For this review, take the finished solid that the model builds, in its own axes (mm). A direction names the side the tool comes from. Coordinates: 2 decimals unless noted, no trailing zeros. Order: outer loops, then holes, each group sorted by start corner. A loop starts at its lowest first (then second) coordinate and runs counter-clockwise, first axis right, second up. Notation, with made-up numbers: (51, 12.25) -> (84, 12.25) arc R33 cw to (84, 45.25) -> close; hole circle Ø1 at (-26.5, -34.5). An arc over 180 degrees is marked (long way). Return JSON: item names as keys, results as strings. Group by question number.
Item 1: Draft analysis for pull direction Z (two halves, no side actions). For faces 3 (the cylindrical face through (-276.009, 3.694, -370.875)), 4 (the flat face through (-111.6, 7.83, -280.08)), 5 (the flat face through (-258, 8, 0)), state which applies: +Z half, -Z half, draft (parallel to the pull), parting line (faces both ways), or undercut.
Item 2: For line 1 along Y through (x, z) = (-252, -378) (3 decimals); line 2 along Z through (x, y) = (-79, 7.75); line 3 along Z through (x, y) = (-194, 1.25), list the stretches that pass through material, from the lowest coordinate up.
Item 3: Take a section at D-D (x = -396.5). Write out the cut boundary in (y, z) (3 decimals).
Item 4: Take a section at B-B (x = -91.5). Write out the cut boundary in (y, z) (3 decimals).
Item 5: Take a section at C-C (z = -192). Write out the cut boundary in (x, y) (3 decimals).
Item 6: Machinability: for faces 1 (the cylindrical face through (-438.72, 3.69, -70.96)), 2 (the flat face through (-536.086, 9.59, -29.327)), which of the approach directions +Z, -Z, +X, -X, +Y, -Y give a long, thin tool a straight path to every point of the face, cutting with its end or side? Answer none if there is none.
Item 7: Take a section at A-A (z = -393.5). Write out the cut boundary in (x, y) (3 decimals), then the cut area to 3 significant figures.
Item 8: Insertion check: pin 1 (10.5 mm diameter, centred on x = -278.11, z = -434.34, fed in from -Y); pin 2 (6 mm diameter, centred on x = -345.5, y = 10, fed in from -Z); pin 3 (4 mm diameter, centred on x = -128, y = 2.5, fed in from -Z); pin 4 (5 mm diameter, centred on x = -502.2, z = -72.44, fed in from +Y). Each pin has a flat end and moves straight along its axis. Give the tip position at first contact, or say it passes through.
```python
from build123d import *

# Parameters (mm, degrees)
BOSS_EXTRUDE1_DEPTH = 15.875
SKETCH2_R           = 3.96875
CUT_EXTRUDE1_DEPTH  = 16.875
SKETCH3_R           = 63.5
SKETCH3_R_2         = 69.85
CUT_EXTRUDE2_DEPTH  = 7.493


with BuildPart() as part:
    # Sketch1 → Boss-Extrude1 (new body)
    with BuildSketch(Plane(origin=(0, 0, 0), x_dir=(1, 0, 0), z_dir=(0, 1, 0))):
        Polygon((0, 0), (-523.875, 0), (-555.849378124, 76.79442277), (-326.138209959, 479.425), (-220.118609959, 479.425), (0, 75.0824), align=None)
    extrude(amount=BOSS_EXTRUDE1_DEPTH)

    # Sketch2 → Cut-Extrude1 (cut, through all)
    with BuildSketch(Plane(origin=(0, 15.875, 0), x_dir=(1, 0, 0), z_dir=(0, 1, 0))):
        with Locations((-278.106809959, 434.34)):
            Circle(SKETCH2_R)
        with Locations((-502.204578124, 72.4408)):
            Circle(SKETCH2_R)
        with Locations((-49.7332, 44.9326)):
            Circle(SKETCH2_R)
    extrude(amount=-CUT_EXTRUDE1_DEPTH, mode=Mode.SUBTRACT)

    # Sketch3 → Cut-Extrude2 (cut)
    with BuildSketch(Plane.XZ):
        with Locations((-502.204578124, -72.4408)):
            Circle(SKETCH3_R)
        with Locations((-49.7332, -44.9326)):
            Circle(SKETCH3_R_2)
        with Locations((-278.106809959, -434.34)):
            Circle(SKETCH3_R)
    extrude(amount=-CUT_EXTRUDE2_DEPTH, mode=Mode.SUBTRACT)


solid = part.part
```
Findings below:
{
 "1": {"face 3": "undercut", "face 4": "-Z half", "face 5": "+Z half"},
 "2": {"line 1": "y = 7.493 to 15.875", "line 2": "z = -220.2 to 0", "line 3": "z = -431.45 to 0"},
 "3": {"outline": "(0, -356.097) -> (15.875, -356.097) -> (15.875, 0) -> (0, 0) -> close"},
 "4": {"outline": "(0, -243.162) -> (15.875, -243.162) -> (15.875, 0) -> (7.493, 0) -> (7.493, -100.92) -> (0, -100.92) -> close"},
 "5": {"outline": "(-490.122, 0) -> (-63.648, 0) -> (-63.648, 15.875) -> (-490.122, 15.875) -> close"},
 "6": {"face 1": "-Y", "face 2": "+Z, -X, +Y, -Y"},
 "7": {"outline": "(-375.161, 0) -> (-326.731, 0) -> (-326.731, 7.493) -> (-229.482, 7.493) -> (-229.482, 0) -> (-173.342, 0) -> (-173.342, 15.875) -> (-375.161, 15.875) -> close", "area": "2,480 mm2"},
 "8": {"pin 1": "stops at y = 7.49", "pin 2": "stops at z = -450.75", "pin 3": "stops at z = -313.88", "pin 4": "passes through"}
}
